```python
from build123d import *

# Parameters (mm, degrees)
SKETCH2_W                          = 75
SKETCH2_H                          = 75
SKETCH2_W_2                        = 57
SKETCH2_H_2                        = 65
BOSS_EXTRUDE1_DEPTH                = 41.91
CUT_EXTRUDE1_DEPTH                 = 92.91
SKETCH6_W                          = 22
SKETCH6_H                          = 6
CUT_EXTRUDE2_DEPTH                 = 92.91
CUT_EXTRUDE3_DEPTH                 = 92.91
CIRPATTERN1_COUNT                  = 4
TAP_DRILL_FOR_6_40_TAP1_AT_2_COUNT = 2
TAP_DRILL_FOR_6_40_TAP1_AT_2_PITCH = 32
CIRPATTERN2_COUNT                  = 2
TAP_DRILL_FOR_6_40_TAP2_AT_2_COUNT = 2
TAP_DRILL_FOR_6_40_TAP2_AT_2_PITCH = 49
CIRPATTERN4_COUNT                  = 2


with BuildPart() as part:
    # Sketch2 → Boss-Extrude1 (new body)
    with BuildSketch(Plane(origin=(0, 0, 0), x_dir=(1, 0, 0), z_dir=(0, 1, 0))):
        with Locations((-5.814990765, -18.037415397)):
            Rectangle(SKETCH2_W, SKETCH2_H)
        with Locations((-5.814990765, -18.037415397)):
            Rectangle(SKETCH2_W_2, SKETCH2_H_2, mode=Mode.SUBTRACT)
    extrude(amount=BOSS_EXTRUDE1_DEPTH)

    # Sketch4 → Cut-Extrude1 (cut)
    with BuildSketch(Plane(origin=(0, 0, -19.462584603), x_dir=(-1, 0, 0), z_dir=(0, 0, -1))):
        Polygon((16.782729205, 41.915021022), (-5.180449965, 41.91), (-5.180449965, 35.91), (16.819550035, 35.91), align=None)
    extrude(amount=-CUT_EXTRUDE1_DEPTH, mode=Mode.SUBTRACT)

    # Sketch6 → Cut-Extrude2 (cut)
    with BuildSketch(Plane.ZY.offset(43.314990765)):
        with Locations((18.037415397, 38.91)):
            Rectangle(SKETCH6_W, SKETCH6_H)
    extrude(amount=-CUT_EXTRUDE2_DEPTH, mode=Mode.SUBTRACT)

    # Sketch7 → Cut-Extrude3 (cut)
    with BuildSketch(Plane(origin=(0, 41.91, 0), x_dir=(1, 0, 0), z_dir=(0, 1, 0))):
        Polygon((31.685009235, 12.996800195), (25.219224828, 19.462584603), (31.685009235, 19.462584603), align=None)
    cut_extrude3 = extrude(amount=-CUT_EXTRUDE3_DEPTH, mode=Mode.SUBTRACT)

    # CirPattern1: Cut-Extrude3 ×4 about axis
    cirpattern1_axis = Axis((-5.814990765, 0, 18.037415397), (0, 1, 0))
    for i in range(1, CIRPATTERN1_COUNT):
        add(cut_extrude3.rotate(cirpattern1_axis, i * 360 / CIRPATTERN1_COUNT), mode=Mode.SUBTRACT)

    # Sketch18 → Tap Drill for _6-40 Tap1 (revolve, cut)
    with BuildSketch(Plane(origin=(-38.814990765, 41.91, 2.037415397), x_dir=(0, 0, 1), z_dir=(1, 0, 0))):
        Polygon((0, 0), (0, 20.862295074), (1.4351, 20), (1.4351, 0), align=None)
    tap_drill_for_6_40_tap1 = revolve(axis=Axis((-38.814990765, 48.26, 2.037415397), (0, -1, 0)), mode=Mode.SUBTRACT)

    # Tap Drill for _6-40 Tap1 at 2: Tap Drill for _6-40 Tap1 ×2
    with Locations(*[(0, 0, i * TAP_DRILL_FOR_6_40_TAP1_AT_2_PITCH) for i in range(1, TAP_DRILL_FOR_6_40_TAP1_AT_2_COUNT)]):
        add(tap_drill_for_6_40_tap1, mode=Mode.SUBTRACT)

    # CirPattern2: Tap Drill for _6-40 Tap1 ×2 about axis
    cirpattern2_axis = Axis((-5.814990765, 0, 18.037415397), (0, 1, 0))
    for i in range(1, CIRPATTERN2_COUNT):
        add(tap_drill_for_6_40_tap1.rotate(cirpattern2_axis, i * 360 / CIRPATTERN2_COUNT), mode=Mode.SUBTRACT)

    # CirPattern2 copy 1 sketch → CirPattern2 copy 1 (revolve, cut)
    with BuildSketch(Plane(origin=(27.185009235, 41.91, 2.037415397), x_dir=(0, 0, -1), z_dir=(-1, 0, 0))):
        Polygon((0, 0), (0, 20.862295074), (1.4351, 20), (1.4351, 0), align=None)
    revolve(axis=Axis((27.185009235, 48.26, 2.037415397), (0, -1, 0)), mode=Mode.SUBTRACT)

    # Sketch23 → Tap Drill for _6-40 Tap2 (revolve, cut)
    with BuildSketch(Plane(origin=(-30.314990765, 41.91, -16.962584603), x_dir=(0, 0, 1), z_dir=(1, 0, 0))):
        Polygon((0, 0), (0, 20.862295074), (1.4351, 20), (1.4351, 0), align=None)
    tap_drill_for_6_40_tap2 = revolve(axis=Axis((-30.314990765, 48.26, -16.962584603), (0, -1, 0)), mode=Mode.SUBTRACT)

    # Tap Drill for _6-40 Tap2 at 2: Tap Drill for _6-40 Tap2 ×2
    with Locations(*[(i * TAP_DRILL_FOR_6_40_TAP2_AT_2_PITCH, 0, 0) for i in range(1, TAP_DRILL_FOR_6_40_TAP2_AT_2_COUNT)]):
        add(tap_drill_for_6_40_tap2, mode=Mode.SUBTRACT)

    # CirPattern4: Tap Drill for _6-40 Tap2 ×2 about axis
    cirpattern4_axis = Axis((-5.814990765, 0, 18.037415397), (0, 1, 0))
    for i in range(1, CIRPATTERN4_COUNT):
        add(tap_drill_for_6_40_tap2.rotate(cirpattern4_axis, i * 360 / CIRPATTERN4_COUNT), mode=Mode.SUBTRACT)

    # CirPattern4 copy 1 sketch → CirPattern4 copy 1 (revolve, cut)
    with BuildSketch(Plane(origin=(-30.314990765, 41.91, 53.037415397), x_dir=(0, 0, -1), z_dir=(-1, 0, 0))):
        Polygon((0, 0), (0, 20.862295074), (1.4351, 20), (1.4351, 0), align=None)
    revolve(axis=Axis((-30.314990765, 48.26, 53.037415397), (0, -1, 0)), mode=Mode.SUBTRACT)


solid = part.part
```
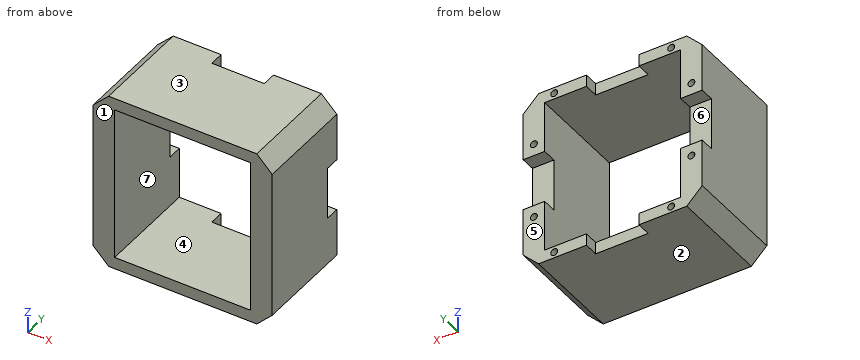
Read the model definition and answer for the solid it produces. Units are mm, in the model's axes. Face numbers are marked on the shaded views. A direction names the side the tool comes from. Give positions to 0.01 mm unless a question says otherwise; leave off trailing zeros. Order: outer loops, then holes, each group sorted by start corner. A loop starts at its lowest first (then second) coordinate and runs counter-clockwise, first axis right, second up.
(1) For the marked faces 5, 6 and 7, determine the directions among +Z, -Z, +X, -X, +Y, -Y from which every point of the face is accessible in a straight line to the end or side of a thin tool.
(2) Straight lines are drawn through the part: L1, parallel to X at y = 5.5, z = -0.5 (3 decimals); L2, parallel to Z at x = -4, y = 24.5; L3, parallel to Z at x = -31, y = 27. For each, find the intervals that lie inside material, in ascending order.
(3) Find section C-C (y = 18). Give the vertices of the cut face in (x, z) (3 decimals), plus the area to 3 significant figures.
(4) Given pin 1 (1.5 mm diameter, centred on y = 40, z = 53, fed in from -X); pin 2 (7 mm diameter, centred on x = -36.5, z = 22.5, fed in from +Y); pin 3 (1.5 mm diameter, centred on y = 40, z = -17.5, fed in from -X), each flat-ended and moving along its own axis, determine where each tip first touches the part or whether it passes through.
(5) Find section D-D (x = 24). Give the vertices of the cut face in (y, z).
(6) Find section A-A (x = -8). Give the vertices of the cut face in (y, z), plus the area to 3 significant figures.
(7) For a pull along Z with two mould halves and no side action, classify the marked faces 1, 2, 3 and 4 as released by +Z, released by -Z, zero draft, split by the parting line, or undercut.
(8) Find section B-B (z = 22.5). Give the vertices of the cut face in (x, y) (3 decimals), plus the area to 3 significant figures.
Result sheet:
1. face 5: +Z, -Z, +X, -X, +Y
1. face 6: +X, -X, +Y
1. face 7: +Y, -Y
2. L1: x = -43.315 to -34.315, 22.685 to 31.685
2. L2: z = -19.46 to -14.46, 50.54 to 55.54
2. L3: z = -19.46 to -18.22, -15.7 to -14.46, 50.54 to 51.78, 54.3 to 55.54
3. outline: (-43.315, -12.997) - (-36.849, -19.463) - (25.219, -19.463) - (31.685, -12.997) - (31.685, 49.072) - (25.219, 55.537) - (-36.849, 55.537) - (-43.315, 49.072) - close; hole (-34.315, -14.463) - (22.685, -14.463) - (22.685, 50.537) - (-34.315, 50.537) - close
3. area: 1,840 mm2
4. pin 1: stops at x = -40.14
4. pin 2: stops at y = 35.91
4. pin 3: stops at x = -39.56
5. outline: (0, -19.46) - (41.91, -19.46) - (41.91, 7.04) - (35.91, 7.04) - (35.91, 29.04) - (41.91, 29.04) - (41.91, 55.54) - (0, 55.54) - close
6. outline: (0, -19.46) - (35.91, -19.46) - (35.91, -14.46) - (0, -14.46) - close; (0, 50.54) - (35.91, 50.54) - (35.91, 55.54) - (0, 55.54) - close
6. area: 359 mm2
7. face 1: zero draft
7. face 2: released by -Z
7. face 3: released by +Z
7. face 4: undercut
8. outline: (-43.315, 0) - (-34.315, 0) - (-34.315, 35.91) - (-43.315, 35.91) - close; (22.685, 0) - (31.685, 0) - (31.685, 35.91) - (22.685, 35.91) - close
8. area: 646 mm2
